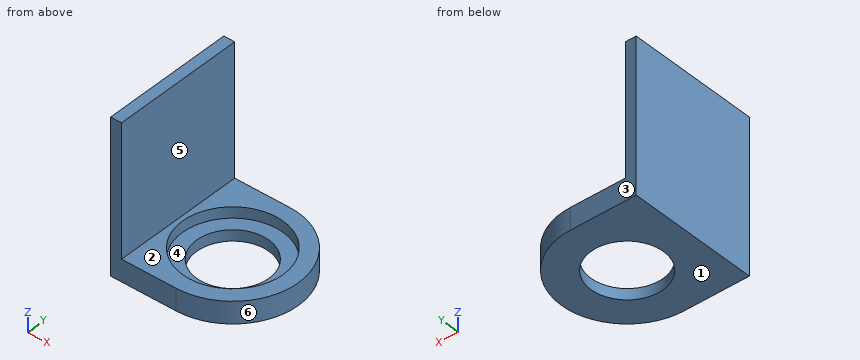
```python
from build123d import *

# Parameters (mm, degrees)
F1_DEPTH = 12.7
F2_R     = 29.21
F3_DEPTH = 6.35
F4_R     = 20.955
F5_DEPTH = 6.35
F6_W     = 6.35
F6_H     = 76.2
F7_DEPTH = 76.2


with BuildPart() as f1:
    # F0 (on Top) → F1 (new body)
    with BuildSketch(Plane.XY):
        with BuildLine():
            ThreePointArc((0, -38.1), (38.1, 0), (0, 38.1))
            Line((0, 38.1), (-38.1, 38.1))
            Line((-38.1, 38.1), (-38.1, -38.1))
            Line((-38.1, -38.1), (0, -38.1))
        make_face()
    extrude(amount=F1_DEPTH)

    # F2 (on face) → F3 (cut)
    with BuildSketch(Plane.XY.offset(12.7)):
        Circle(F2_R)
    extrude(amount=-F3_DEPTH, mode=Mode.SUBTRACT)

    # F4 (on face) → F5 (cut)
    with BuildSketch(Plane.XY.offset(6.35)):
        Circle(F4_R)
    extrude(amount=-F5_DEPTH, mode=Mode.SUBTRACT)

    # F6 (on face) → F7 (join)
    with BuildSketch(Plane.XY.offset(12.7)):
        with Locations((-34.925, 0)):
            Rectangle(F6_W, F6_H)
    extrude(amount=F7_DEPTH)


solid = f1.part
```
CAD build for the part. Positions are in the model's coordinates, mm. Face numbers are marked on the shaded views. A direction names the side the tool comes from. Coordinates: 2 decimals unless noted, no trailing zeros. Order: outer loops, then holes, each group sorted by start corner. A loop starts at its lowest first (then second) coordinate and runs counter-clockwise, first axis right, second up. Notation, with made-up numbers: (0, 57) -> (56, 57) arc R7 cw to (56, 61) -> close; hole circle Ø3 at (-19.5, 16.25). An arc over 180 degrees is marked (long way). Use one line per item in the form item = value. Start each with the question number.
1) Band-saw the part on C-C on z = 8. Give the cut face in (x, y), then the cut area to 3 significant figures.
2) Band-saw the part on D-D on x = -10. Give the cut face in (y, z) (3 decimals).
3) Pull direction Y, two halves, no side cores. Call the marked faces 3, 4, 5 and 6: +Y half, -Y half, draft (parallel to the pull), parting line (faces both ways), or undercut.
4) Band-saw the part on B-B on x = 19. Give the cut face in (y, z).
5) Drill centre lines: L1, parallel to Y at x = 0, z = 8; L2, parallel to X at y = -21.5, z = 67; L3, parallel to Z at x = -23, y = -30.5. Where is each one in solid material? Low to high. Write a range as [from, to].
6) Drop flat-ended pins along their axis: pin 1 (6 mm diameter, centred on y = 18.5, z = 66.5, fed in from +X); pin 2 (5 mm diameter, centred on x = 30, y = 9.5, fed in from -Z); pin 3 (2 mm diameter, centred on x = 24.5, y = -15, fed in from +Z). Give the stop position or say it passes through.
7) Tool access for the marked faces 1 and 2: list every direction of +Z, -Z, +X, -X, +Y, -Y with a clear straight run to the whole face (end or side of a thin tool).
8) Band-saw the part on A-A on y = 0. Give the cut face in (x, z) (3 decimals).
Entries:
q1.outline = (-38.1, -38.1) -> (0, -38.1) arc R38.1 ccw to (0, 38.1) -> (-38.1, 38.1) -> close; hole circle Ø58.42 at (0, 0)
q1.area = 2,500 mm2
q2.outline = (-38.1, 0) -> (-18.415, 0) -> (-18.415, 6.35) -> (-27.445, 6.35) -> (-27.445, 12.7) -> (-38.1, 12.7) -> close; (18.415, 0) -> (38.1, 0) -> (38.1, 12.7) -> (27.445, 12.7) -> (27.445, 6.35) -> (18.415, 6.35) -> close
q3.face_3 = +Y half
q3.face_4 = undercut
q3.face_5 = draft
q3.face_6 = parting line
q4.outline = (-33.02, 0) -> (-8.84, 0) -> (-8.84, 6.35) -> (-22.19, 6.35) -> (-22.19, 12.7) -> (-33.02, 12.7) -> close; (8.84, 0) -> (33.02, 0) -> (33.02, 12.7) -> (22.19, 12.7) -> (22.19, 6.35) -> (8.84, 6.35) -> close
q5.L1 = [-38.1, -29.21], [29.21, 38.1]
q5.L2 = [-38.1, -31.75]
q5.L3 = [0, 12.7]
q6.pin_1 = -31.75
q6.pin_2 = 0
q6.pin_3 = 12.7
q7.face_1 = -Z, +X, -X, +Y, -Y
q7.face_2 = +Z, +X, +Y, -Y
q8.outline = (-38.1, 0) -> (-20.955, 0) -> (-20.955, 6.35) -> (-29.21, 6.35) -> (-29.21, 12.7) -> (-31.75, 12.7) -> (-31.75, 88.9) -> (-38.1, 88.9) -> close; (20.955, 0) -> (38.1, 0) -> (38.1, 12.7) -> (29.21, 12.7) -> (29.21, 6.35) -> (20.955, 6.35) -> close
